from build123d import *

# Parameters (mm, degrees)
SKETCH1_R           = 21.75
SKETCH1_R_2         = 19
BOSS_EXTRUDE1_DEPTH = 295
BOSS_EXTRUDE2_REACH = 51.786
SKETCH5_R           = 7
SKETCH5_R_2         = 4
BOSS_EXTRUDE3_REACH = 51.455
SKETCH6_R           = 7
SKETCH6_R_2         = 4
SKETCH7_R           = 4
CUT_EXTRUDE1_DEPTH  = 10
SKETCH8_R           = 4
CUT_EXTRUDE2_DEPTH  = 20


with BuildPart() as part:
    # Sketch1 → Boss-Extrude1 (new body)
    with BuildSketch(Plane(origin=(0, 0, 0), x_dir=(0, 0, -1), z_dir=(1, 0, 0))):
        Circle(SKETCH1_R)
        Circle(SKETCH1_R_2, mode=Mode.SUBTRACT)
    extrude(amount=BOSS_EXTRUDE1_DEPTH)

    # Sketch5 → Boss-Extrude2 (add, up to next)
    with BuildSketch(Plane(origin=(0.022625841, 23.166571161, 5.264124015), x_dir=(0.999999546, -0.000927561, -0.00021607), z_dir=(-0.000952381, -0.975141562, -0.221580746)), mode=Mode.PRIVATE) as boss_extrude2_sk1:
        with Locations((260.436740743, 0.291462923)):
            Circle(SKETCH5_R)
        with Locations((260.436740743, 0.291462923)):
            Circle(SKETCH5_R_2, mode=Mode.SUBTRACT)
    boss_extrude2_tool1 = extrude(boss_extrude2_sk1.sketch, amount=BOSS_EXTRUDE2_REACH, mode=Mode.PRIVATE) - part.part
    add(boss_extrude2_tool1.solids().sort_by_distance((253.657243, 22.866727, 5.493539))[0])

    # Sketch6 → Boss-Extrude3 (add, up to next)
    with BuildSketch(Plane(origin=(0.192055035, 27.157330053, -0.682085947), x_dir=(0.999975011, -0.007067306, 0.000177503), z_dir=(-0.007069535, -0.999659759, 0.025107545)), mode=Mode.PRIVATE) as boss_extrude3_sk1:
        with Locations((105.278439441, 0.08752168)):
            Circle(SKETCH6_R)
        with Locations((105.278439441, 0.08752168)):
            Circle(SKETCH6_R_2, mode=Mode.SUBTRACT)
    boss_extrude3_tool1 = extrude(boss_extrude3_sk1.sketch, amount=BOSS_EXTRUDE3_REACH, mode=Mode.PRIVATE) - part.part
    add(boss_extrude3_tool1.solids().sort_by_distance((98.666024, 26.463564, -0.577112))[0])

    # Sketch7 → Cut-Extrude1 (cut)
    with BuildSketch(Plane(origin=(0.022625841, 23.166571161, 5.264124015), x_dir=(0.999999546, -0.000927561, -0.00021607), z_dir=(0.000952381, 0.975141562, 0.221580746))):
        with Locations((260.436740743, -0.291462923)):
            Circle(SKETCH7_R)
    extrude(amount=-CUT_EXTRUDE1_DEPTH, mode=Mode.SUBTRACT)

    # Sketch8 → Cut-Extrude2 (cut)
    with BuildSketch(Plane(origin=(0.192055035, 27.157330053, -0.682085947), x_dir=(0.999975011, -0.007067306, 0.000177503), z_dir=(0.007069535, 0.999659759, -0.025107545))):
        with Locations((105.278439441, -0.08752168)):
            Circle(SKETCH8_R)
    extrude(amount=-CUT_EXTRUDE2_DEPTH, mode=Mode.SUBTRACT)


solid = part.part
Part model, mm, in its own coordinate system. Round coordinates to 2 decimals unless told otherwise and drop trailing zeros. Loops run counter-clockwise (first coordinate to the right, second up) from the corner with the lowest first, then second, coordinate; pieces in that order, holes last. Notation, with made-up numbers: (3.5, 3.25) - (40.5, 3.25) arc R9 ccw to (40.5, 10.25) - close; hole circle Ø4 at (-25, 52.5). An arc over 180 degrees is marked (long way). Answer as a JSON object with one key per item and string values.
Item 1: Band-saw the part on A-A on y = 0. List the corners of the cut face in (x, z), plus the area to 3 significant figures.
Output:
{"outline": "(0, -21.75) - (295, -21.75) - (295, -19) - (0, -19) - close; (0, 19) - (295, 19) - (295, 21.75) - (0, 21.75) - close", "area": "1,620 mm2"}
Item 2: Pull direction Y, two halves, no side cores. Call faces 1 (the face through (145.435, -16.856, -8.767)), 2 (the face through (264.2, 20.4, 11)): pulls with the +Y half, pulls with the -Y half, needs draft (parallel to the pull), parting line crosses it, or undercut.
Output:
{"face 1": "undercut", "face 2": "undercut"}
Item 3: Band-saw the part on C-C on y = -12. List the corners of the cut face in (x, z).
Output:
{"outline": "(0, -18.14) - (295, -18.14) - (295, -14.73) - (0, -14.73) - close; (0, 14.73) - (295, 14.73) - (295, 18.14) - (0, 18.14) - close"}
Item 4: Pin check, flat tips, straight feed: pin 1 (12 mm diameter, centred on x = 261, z = 1.5, fed in from +Y); pin 2 (10 mm diameter, centred on x = 107, z = 4, fed in from +Y); pin 3 (3 mm diameter, centred on x = 191, y = -6.5, fed in from +Z); pin 4 (1 mm diameter, centred on x = 197, z = 13.5, fed in from -Y). Stop position of each tip, or through.
Output:
{"pin 1": "y = 24.41", "pin 2": "y = 26.6", "pin 3": "z = 21.17", "pin 4": "y = -17.44"}
Item 5: Wall check: L1, parallel to X at y = 22, z = 6; L2, parallel to Y at x = 217, z = 0; L3, parallel to Z at x = 265.5, y = 2. Give the ranges that are in metal, low to high.
Output:
{"L1": "102.75 to 108.12, 253.49 to 256.52, 264.4 to 267.42", "L2": "-21.75 to -19, 19 to 21.75", "L3": "-21.66 to -18.89, 18.89 to 21.66"}
Item 6: Band-saw the part on B-B on x = 83. List the corners of the cut face in (y, z).
Output:
{"outline": "circle Ø43.5 at (0, 0); hole circle Ø38 at (0, 0)"}
